Input: part model. Units: mm. Frame: model coordinates. Face numbers are marked on the shaded views. Round coordinates to 2 decimals unless told otherwise and drop trailing zeros. Loops run counter-clockwise (first coordinate to the right, second up) from the corner with the lowest first, then second, coordinate; pieces in that order, holes last.
(1) Draft query along X for the marked faces 1, 2 and 3. Return one class per face: released by +X, released by -X, zero draft, split by the parting line, or undercut.
(2) Cut plane C-C, the plane y = -1. Output: boundary loops of the cut face in (x, z) (3 decimals).
(3) Cut plane A-A, the plane z = 0.1. Output: boundary loops of the cut face in (x, y) (3 decimals), and give its area (3 significant figures).
(4) First-contact query: pin 1 Ø2 at (x, y) = (0.5, -3.5) entering from +Z; pin 2 Ø0.7 at (y, z) = (-3.5, 0.5) entering from -X; pin 3 Ø0.5 at (x, y) = (-1.5, -3.5) entering from +Z. Flat tips, straight axial feed; report the tip coordinate or a pass-through.
(5) Cut plane B-B, the plane x = 1.75. Output: boundary loops of the cut face in (y, z), and give its area (3 significant figures).
(6) Line query: line 1 (X direction, y = -4, z = 0.1); line 2 (Y direction, x = 0.05, z = 0.8); line 3 (Z direction, x = -1.75, y = 1.75). Output: solid intervals per line, ascending.
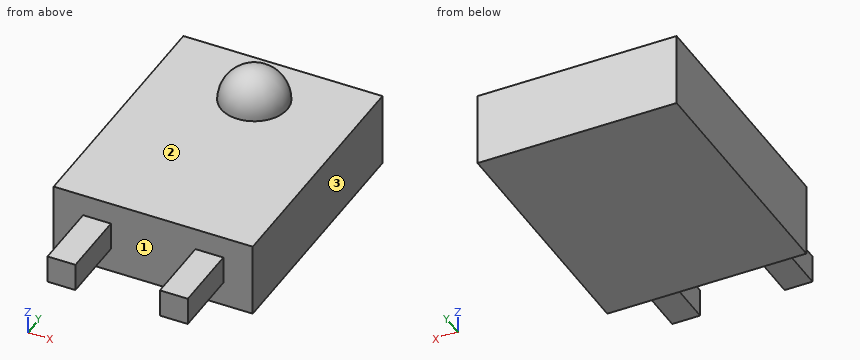
from build123d import *

# Parameters (mm, degrees)
BOSS_EXTRUDE1_DEPTH      = 1.14
BOSS_EXTRUDE1_DEPTH_BACK = 0.56
SKETCH2_W                = 4.57
SKETCH2_H                = 5.84
SKETCH3_R                = 0.76
BOSS_EXTRUDE2_DEPTH      = 0.76
FILLET1_R                = 0.76
SKETCH4_W                = 0.64
SKETCH4_H                = 0.64
BOSS_EXTRUDE3_DEPTH      = 1.6
SKETCH5_W                = 0.64
SKETCH5_H                = 0.64
BOSS_EXTRUDE4_DEPTH      = 1.6


with BuildPart() as part:
    # Sketch2 → Boss-Extrude1 (new, two sides: drawn at the far end of the back side and taken through both)
    with BuildSketch(Plane.XY.offset(-BOSS_EXTRUDE1_DEPTH_BACK)):
        Rectangle(SKETCH2_W, SKETCH2_H)
    extrude(amount=BOSS_EXTRUDE1_DEPTH + BOSS_EXTRUDE1_DEPTH_BACK)

    # Sketch3 → Boss-Extrude2 (add)
    with BuildSketch(Plane.XY.offset(1.14)):
        with Locations(Location((0, 1.63, 0), (0, 0, 180))):
            Circle(SKETCH3_R)
    extrude(amount=BOSS_EXTRUDE2_DEPTH)

    # Fillet1
    fillet1_edges = [part.edges().sort_by_distance(p)[0] for p in [
        (0.76, 1.63, 1.9),
    ]]
    fillet(fillet1_edges, radius=FILLET1_R - 0.0001)  # a hair under: the kernel refuses the full size

    # Sketch4 → Boss-Extrude3 (add)
    with BuildSketch(Plane.XZ.offset(2.92)):
        with Locations((1.29, 0.32)):
            Rectangle(SKETCH4_W, SKETCH4_H)
    extrude(amount=BOSS_EXTRUDE3_DEPTH)

    # Sketch5 → Boss-Extrude4 (add)
    with BuildSketch(Plane.XZ.offset(2.92)):
        with Locations((-1.29, 0.32)):
            Rectangle(SKETCH5_W, SKETCH5_H)
    extrude(amount=BOSS_EXTRUDE4_DEPTH)


solid = part.part
Reported:
1. face 1: undercut
1. face 2: zero draft
1. face 3: released by +X
2. outline: (-2.285, -0.56) - (2.285, -0.56) - (2.285, 1.14) - (-2.285, 1.14) - close
3. outline: (-2.285, -2.92) - (-1.61, -2.92) - (-1.61, -4.52) - (-0.97, -4.52) - (-0.97, -2.92) - (0.97, -2.92) - (0.97, -4.52) - (1.61, -4.52) - (1.61, -2.92) - (2.285, -2.92) - (2.285, 2.92) - (-2.285, 2.92) - close
3. area: 28.7 mm2
4. pin 1: stops at z = 1.14
4. pin 2: stops at x = -1.61
4. pin 3: stops at z = 0.64
5. outline: (-2.92, -0.56) - (2.92, -0.56) - (2.92, 1.14) - (-2.92, 1.14) - close
5. area: 9.93 mm2
6. line 1: x = -1.61 to -0.97, 0.97 to 1.61
6. line 2: y = -2.92 to 2.92
6. line 3: z = -0.56 to 1.14
